```python
from build123d import *

# Parameters (mm, degrees)
SKICA1_W                 = 54.6
SKICA1_H                 = 54.6
P_IDAT_VYSUNUT_M2_DEPTH  = 3
SKICA4_W                 = 25
SKICA4_H                 = 5
ODEBRAT_VYSUNUT_M1_DEPTH = 2
SKICA5_W                 = 54.6
SKICA5_H                 = 5
ODEBRAT_VYSUNUT_M3_DEPTH = 1
SKICA10_W                = 5
SKICA10_H                = 10
P_IDAT_VYSUNUT_M6_DEPTH  = 10
ODEBRAT_VYSUNUT_M6_DEPTH = 10
P_IDAT_VYSUNUT_M9_DEPTH  = 15
SKICA17_R                = 2
ODEBRAT_VYSUNUT_M8_DEPTH = 4
SKICA19_W                = 7.8
SKICA19_H                = 7.8
P_IDAT_VYSUNUT_M10_DEPTH = 18
SKICA20_R                = 2.4
ODEBRAT_VYSUNUT_M9_DEPTH = 1.7
ZAOBLIT1_R               = 3


with BuildPart() as part:
    # Skica1 → Přidat vysunutím2 (new body)
    with BuildSketch(Plane.XY):
        Rectangle(SKICA1_W, SKICA1_H)
    extrude(amount=P_IDAT_VYSUNUT_M2_DEPTH)

    # Skica4 → Odebrat vysunutím1 (cut)
    with BuildSketch(Plane.XY.offset(3)):
        Rectangle(SKICA4_W, SKICA4_H)
    extrude(amount=-ODEBRAT_VYSUNUT_M1_DEPTH, mode=Mode.SUBTRACT)

    # Skica5 → Odebrat vysunutím3 (cut)
    with BuildSketch(Plane(origin=(0, 0, 0), x_dir=(-1, 0, 0), z_dir=(0, 0, -1))):
        Rectangle(SKICA5_W, SKICA5_H)
    extrude(amount=-ODEBRAT_VYSUNUT_M3_DEPTH, mode=Mode.SUBTRACT)

    # Skica10 → Přidat vysunutím6 (add)
    with BuildSketch(Plane.XY.offset(3)):
        with Locations((-20.5, 0)):
            Rectangle(SKICA10_W, SKICA10_H)
        with Locations((20.5, 0)):
            Rectangle(SKICA10_W, SKICA10_H)
    extrude(amount=P_IDAT_VYSUNUT_M6_DEPTH)

    # Skica12 → Odebrat vysunutím6 (cut)
    with BuildSketch(Plane(origin=(0, 5, 0), x_dir=(1, 0, 0), z_dir=(0, 1, 0))):
        Polygon((-18, -13), (-18, -11), (-19.5, -12), align=None)
        Polygon((18, -13), (18, -11), (19.5, -12), align=None)
    extrude(amount=-ODEBRAT_VYSUNUT_M6_DEPTH, mode=Mode.SUBTRACT)

    # Skica14 → Přidat vysunutím9 (add)
    with BuildSketch(Plane.XY.offset(3)):
        Polygon((27.3, 27.3), (-27.3, 27.3), (-27.3, -27.3), (-26.3, -27.3), (-26.3, 26.3), (26.3, 26.3), (26.3, -27.3), (27.3, -27.3), align=None)
    extrude(amount=P_IDAT_VYSUNUT_M9_DEPTH)

    # Skica17 → Odebrat vysunutím8 (cut)
    with BuildSketch(Plane(origin=(0, 0, 1), x_dir=(-1, 0, 0), z_dir=(0, 0, -1))):
        with Locations((-20.3, 0)):
            Circle(SKICA17_R)
        with Locations((20.3, 0)):
            Circle(SKICA17_R)
    extrude(amount=-ODEBRAT_VYSUNUT_M8_DEPTH, mode=Mode.SUBTRACT)

    # Skica19 → Přidat vysunutím10 (add)
    with BuildSketch(Plane(origin=(0, 0, 0), x_dir=(-1, 0, 0), z_dir=(0, 0, -1))):
        with Locations((-23.4, 23.4)):
            Rectangle(SKICA19_W, SKICA19_H)
        with Locations((23.4, 23.4)):
            Rectangle(SKICA19_W, SKICA19_H)
        with Locations((-23.4, -23.4)):
            Rectangle(SKICA19_W, SKICA19_H)
        with Locations((23.4, -23.4)):
            Rectangle(SKICA19_W, SKICA19_H)
    extrude(amount=-P_IDAT_VYSUNUT_M10_DEPTH)

    # Skica20 → Odebrat vysunutím9 (cut)
    with BuildSketch(Plane.XY.offset(18)):
        with Locations((-23.4, -23.4)):
            Circle(SKICA20_R)
        with Locations((-23.4, 23.4)):
            Circle(SKICA20_R)
        with Locations((23.400280565, 23.4)):
            Circle(SKICA20_R)
        with Locations((23.400280565, -23.4)):
            Circle(SKICA20_R)
    extrude(amount=-ODEBRAT_VYSUNUT_M9_DEPTH, mode=Mode.SUBTRACT)

    # Zaoblit1
    zaoblit1_edges = [part.edges().sort_by_distance(p)[0] for p in [
        (19.5, 19.5, 10.5),
        (-19.5, 19.5, 10.5),
        (19.5, -19.5, 10.5),
        (-19.5, -19.5, 10.5),
    ]]
    fillet(zaoblit1_edges, radius=ZAOBLIT1_R)


solid = part.part
```
CAD build for the part. Positions are in the model's coordinates, mm. A direction names the side the tool comes from. Round coordinates to 2 decimals unless told otherwise and drop trailing zeros. Loops run counter-clockwise (first coordinate to the right, second up) from the corner with the lowest first, then second, coordinate; pieces in that order, holes last. Notation, with made-up numbers: M 10.5,54.25 L 40.5,54.25 A12 cw 40.5,69.25 Z; hole C 45,22.25 d8. An arc over 180 degrees is marked long. Return JSON: item names as keys, results as strings. Group by question number.
(1) Mould opens along X. For faces 5 (the flat face through (-19.5, -25, 10)), 6 (the flat face through (0, 15, 0)) say: +X half, -X half, draft (parallel to the pull), parting line (faces both ways), or undercut.
(2) Saw through at C-C, the plane z = 6.5. List the corners of the cut face in (x, y), and give its area (3 significant figures).
(3) Saw through at B-B, the plane x = 3.5. List the corners of the cut face in (y, z).
(4) Tool access for faces 1 (the flat face through (12.5, 0, 2)), 2 (the flat face through (18, -1, 1)), 3 (the flat face through (26.3, 0, 10)), 4 (the cylindrical face through (18.453, -0.766, 2.972)): list every direction of +Z, -Z, +X, -X, +Y, -Y with a clear straight run to the whole face (end or side of a thin tool).
(5) Saw through at D-D, the plane y = 23.4. List the corners of the cut face in (x, z).
(6) Wall check: probe 1 along Y at (x, z) = (-23.4, 17.5); probe 2 along X at (y, z) = (15, 9.75); probe 3 along X at (y, z) = (23, 15). Give the ranges that are in metal, low to high. Write a range as [from, to].
(7) Drop flat-ended pins along their axis: P1, Ø1.4, axis at x = -23, y = 24.5, coming from the +Z side; P2, Ø4.5, axis at x = -6, z = 8, coming from the -Y side; P3, Ø6, axis at x = -3.5, y = -2.5, coming from the +Z side. Give the stop position or say it passes through.
Answer list:
{
 "1": {"face 5": "undercut", "face 6": "draft"},
 "2": {"outline": "M -27.3,-27.3 L -19.5,-27.3 L -19.5,-22.5 A3 ccw -22.5,-19.5 L -26.3,-19.5 L -26.3,19.5 L -22.5,19.5 A3 ccw -19.5,22.5 L -19.5,26.3 L 19.5,26.3 L 19.5,22.5 A3 ccw 22.5,19.5 L 26.3,19.5 L 26.3,-19.5 L 22.5,-19.5 A3 ccw 19.5,-22.5 L 19.5,-27.3 L 27.3,-27.3 L 27.3,27.3 L -27.3,27.3 Z; M -23,-5 L -18,-5 L -18,5 L -23,5 Z; M 18,-5 L 23,-5 L 23,5 L 18,5 Z", "area": "453 mm2"},
 "3": {"outline": "M -27.3,0 L -2.5,0 L -2.5,3 L -27.3,3 Z; M 2.5,0 L 27.3,0 L 27.3,18 L 26.3,18 L 26.3,3 L 2.5,3 Z"},
 "4": {"face 1": "+Z, -Z", "face 2": "-Z, +X, -X", "face 3": "+Z", "face 4": "-Z"},
 "5": {"outline": "M -27.3,0 L 27.3,0 L 27.3,18 L 25.8,18 L 25.8,16.3 L 21,16.3 L 21,18 L 19.5,18 L 19.5,3 L -19.5,3 L -19.5,18 L -21,18 L -21,16.3 L -25.8,16.3 L -25.8,18 L -27.3,18 Z"},
 "6": {"probe 1": "[-27.3, -25.8], [-21, -19.5], [19.5, 21], [25.8, 27.3]", "probe 2": "[-27.3, -26.3], [26.3, 27.3]", "probe 3": "[-27.3, -19.5], [19.5, 27.3]"},
 "7": {"P1": "z = 16.3", "P2": "y = 26.3", "P3": "z = 3"}
}
